Read the model definition and answer for the solid it produces. Units are mm, in the model's axes. Face numbers are marked on the shaded views. A direction names the side the tool comes from. Give positions to 0.01 mm unless a question says otherwise; leave off trailing zeros. Loops run counter-clockwise (first coordinate to the right, second up) from the corner with the lowest first, then second, coordinate; pieces in that order, holes last.
(1) Which of the six approach directions +Z, -Z, +X, -X, +Y, -Y give full straight-line access (tool end or side, diameter ignored) to the marked faces 1, 2 and 3?
(2) Find section B-B, the plane x = -7. Write down the section's boundary in (y, z), then the cut area to 3 significant figures.
(3) Find section C-C, the plane y = -10. Write down the section's boundary in (x, z), then the cut area to 3 significant figures.
(4) Each of these flat-tipped pins is pushed along its axis until it touches: P1, Ø1, axis at x = 17, z = -3, coming from the -Y side; P2, Ø1.5, axis at x = -39.5, z = 2, coming from the -Y side; P3, Ø4.5, axis at x = 0, z = 2.5, coming from the +Y side; P4, Ø10, axis at x = 4.5, y = 10.5, coming from the -Z side. Where does it stop, or does it pass through?
(5) Straight lines are drawn through the part: probe 1 along Y at (x, z) = (-14.5, -1.5); probe 2 along X at (y, z) = (10, -0.75); probe 3 along X at (y, z) = (-3.5, -2.5). For each, find the intervals that lie inside material, in ascending order.
```python
from build123d import *

# Parameters (mm, degrees)
BOSS_EXTRUDE1_DEPTH = 7.5


with BuildPart() as part:
    # Sketch1 → Boss-Extrude1 (new, symmetric)
    with BuildSketch(Plane.XY):
        with BuildLine():
            Line((-50, 2.5), (-50, 18.5))
            ThreePointArc((-50, 18.5), (-49.707106781, 19.207106781), (-49, 19.5))
            Line((-49, 19.5), (-45, 19.5))
            Line((-45, 19.5), (-43, 19.5))
            ThreePointArc((-43, 19.5), (-42.292893219, 19.207106781), (-42, 18.5))
            Line((-42, 18.5), (-42, 17.5))
            ThreePointArc((-42, 17.5), (-42.292893219, 16.792893219), (-43, 16.5))
            Line((-43, 16.5), (-44, 16.5))
            ThreePointArc((-44, 16.5), (-44.707106781, 16.207106781), (-45, 15.5))
            Line((-45, 15.5), (-45, 7.5))
            ThreePointArc((-45, 7.5), (-44.707106781, 6.792893219), (-44, 6.5))
            Line((-44, 6.5), (-38, 6.5))
            ThreePointArc((-38, 6.5), (-37.292893219, 6.207106781), (-37, 5.5))
            Line((-37, 5.5), (-37, 3.5))
            ThreePointArc((-37, 3.5), (-36.707106781, 2.792893219), (-36, 2.5))
            Line((-36, 2.5), (49, 2.5))
            ThreePointArc((49, 2.5), (49.707106781, 2.207106781), (50, 1.5))
            Line((50, 1.5), (50, -1.5))
            ThreePointArc((50, -1.5), (49.707106781, -2.207106781), (49, -2.5))
            Line((49, -2.5), (-36, -2.5))
            ThreePointArc((-36, -2.5), (-36.707106781, -2.792893219), (-37, -3.5))
            Line((-37, -3.5), (-37, -5.5))
            ThreePointArc((-37, -5.5), (-37.292893219, -6.207106781), (-38, -6.5))
            Line((-38, -6.5), (-41, -6.5))
            ThreePointArc((-41, -6.5), (-41.707106781, -6.792893219), (-42, -7.5))
            Line((-42, -7.5), (-42, -13.5))
            ThreePointArc((-42, -13.5), (-42.292893219, -14.207106781), (-43, -14.5))
            Line((-43, -14.5), (-49, -14.5))
            ThreePointArc((-49, -14.5), (-49.707106781, -14.207106781), (-50, -13.5))
            Line((-50, -13.5), (-50, -12.5))
            ThreePointArc((-50, -12.5), (-49.707106781, -11.792893219), (-49, -11.5))
            Line((-49, -11.5), (-47, -11.5))
            Line((-47, -11.5), (-47, -6.5))
            Line((-47, -6.5), (-49, -6.5))
            ThreePointArc((-49, -6.5), (-49.707106781, -6.207106781), (-50, -5.5))
            Line((-50, -5.5), (-50, -2.5))
            Line((-50, -2.5), (-50, 2.5))
        make_face()
    extrude(amount=BOSS_EXTRUDE1_DEPTH, both=True)


solid = part.part
```
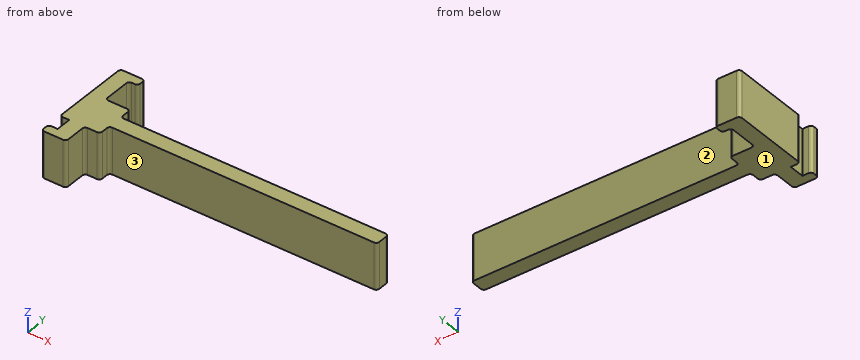
Entries:
1. face 1: -Z, +X, -X, +Y, -Y
1. face 2: +Z, -Z, +X, +Y
1. face 3: +Z, -Z, +X, -Y
2. outline: (-2.5, -7.5) - (2.5, -7.5) - (2.5, 7.5) - (-2.5, 7.5) - close
2. area: 75.0 mm2
3. outline: (-47, -7.5) - (-42, -7.5) - (-42, 7.5) - (-47, 7.5) - close
3. area: 75.0 mm2
4. P1: stops at y = -2.5
4. P2: stops at y = -6.5
4. P3: stops at y = 2.5
4. P4: passes through
5. probe 1: y = -2.5 to 2.5
5. probe 2: x = -50 to -45
5. probe 3: x = -50 to -37
